from build123d import *

# Parameters (mm, degrees)
F0_R     = 22
F1_DEPTH = 50


# Not quite as in the source:
# - a feature names something its author has since deleted; it is built from what else it names


with BuildPart() as f1:
    # F0 (on Front) → F1 (new body)
    with BuildSketch(Plane.XZ):
        Polygon((82.7246823907, 255.5227107533), (-77.2753176093, 255.5227107533), (-77.2753176093, -145.831789898), (-37.2753176093, -645.831789898), (42.6163223386, -645.831789898), (82.7246823907, -144.4772892467), align=None)
        with Locations((2.7246823907, -4.4772892467)):
            Circle(F0_R, mode=Mode.SUBTRACT)
    extrude(amount=F1_DEPTH)


solid = f1.part
Geometry: final body of the model. Coordinates: model frame, mm. Give positions to 0.01 mm unless a question says otherwise; leave off trailing zeros. Loops run counter-clockwise (first coordinate to the right, second up) from the corner with the lowest first, then second, coordinate; pieces in that order, holes last. Notation, with made-up numbers: (71, 2) - (76, 2) arc R32 cw to (76, 30) - close; hole circle Ø1 at (-27, -34). An arc over 180 degrees is marked (long way). Answer as CSV lines item,"result". Start each with the question number.
1. Section C-C, the plane z = -201.5. Return loops of the section in (x, y), plus the area to 3 significant figures.
2. Section B-B, the plane y = -37. Return loops of the section in (x, z).
3. Section D-D, the plane x = 55.5. Return loops of the section in (y, z), plus the area to 3 significant figures.
4. Pin query (flat end, axial travel): P1, Ø6, axis at y = -35, z = -488, coming from the -X side; P2, Ø1.5, axis at y = -11, z = -279.5, coming from the -X side. Return the tip coordinate at first contact, or that it passes through.
5. Ray query, L1, parallel to Z at x = 10, y = -35; L2, parallel to Z at x = 8, y = -45; L3, parallel to X at y = -26.5, z = -304. Return the intervals inside material, ascending.
6. Section A-A, the plane x = -3. Return loops of the section in (y, z), plus the area to 3 significant figures.
7. Draft query along Z for faces 1 (the face through (4, -25, 255.523)), 2 (the face through (82.725, -25, 53)), 3 (the face through (-2.044, -24.65, -25.954)). Return one class per face: released by +Z, released by -Z, zero draft, split by the parting line, or undercut.
Answers:
1,outline,"(-72.82, -50) - (78.16, -50) - (78.16, 0) - (-72.82, 0) - close"
1,area,"7,550 mm2"
2,outline,"(-77.28, -145.83) - (-37.28, -645.83) - (42.62, -645.83) - (82.72, -144.48) - (82.72, 255.52) - (-77.28, 255.52) - close; hole circle Ø44 at (2.72, -4.48)"
3,outline,"(-50, -484.79) - (0, -484.79) - (0, 255.52) - (-50, 255.52) - close"
3,area,"37,000 mm2"
4,P1,"stops at x = -50.14"
4,P2,"stops at x = -66.64"
5,L1,"z = -645.83 to -25.24, 16.28 to 255.52"
5,L2,"z = -645.83 to -25.84, 16.88 to 255.52"
5,L3,"x = -64.62 to 69.96"
6,outline,"(-50, -645.83) - (0, -645.83) - (0, -25.72) - (-50, -25.72) - close; (-50, 16.76) - (0, 16.76) - (0, 255.52) - (-50, 255.52) - close"
6,area,"42,900 mm2"
7,face 1,"released by +Z"
7,face 2,"zero draft"
7,face 3,"undercut"
